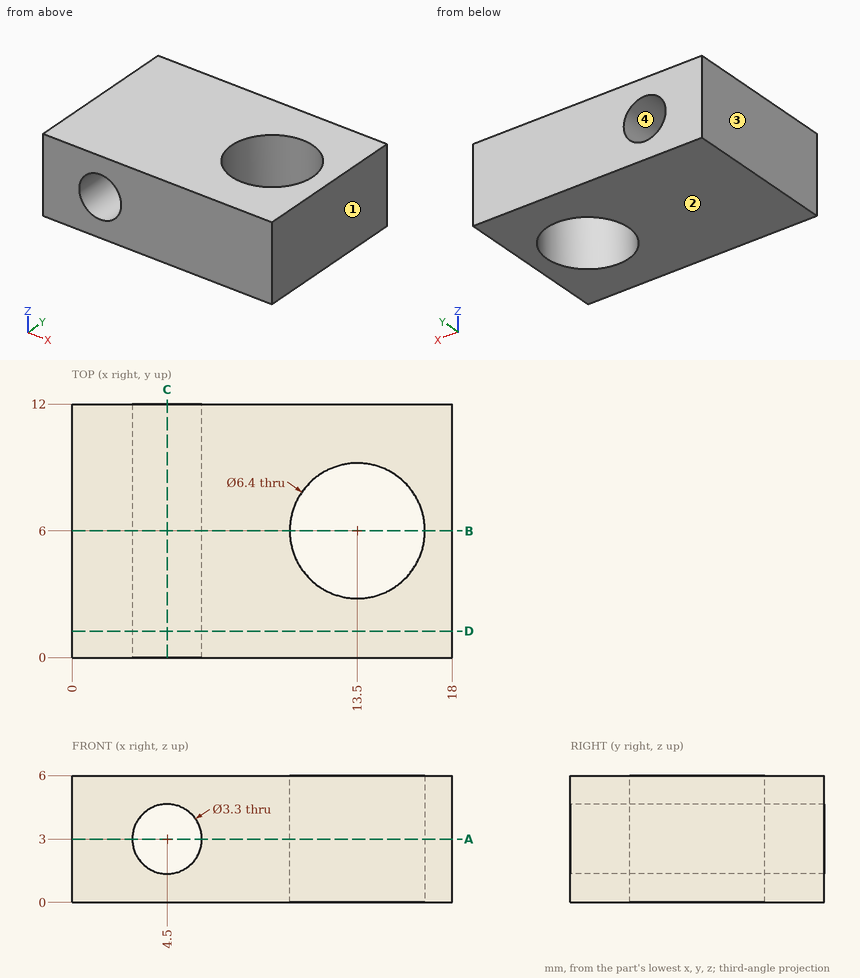
Could you check a few things on this drawing? It's one solid part, dimensions in mm from its lowest x, y, z. Coordinates: 2 decimals unless noted, no trailing zeros. Order: outer loops, then holes, each group sorted by start corner. A loop starts at its lowest first (then second) coordinate and runs counter-clockwise, first axis right, second up. Notation, with made-up numbers: (41.25, 64) - (59.25, 64) arc R22 cw to (59.25, 83) - close; hole circle Ø8 at (52.5, 64.5). An arc over 180 degrees is marked (long way). One line per question, with ' | ' between items. Start each with the question number.
1. If we mould it in two halves opening along X, with no side actions, what happens to the marked faces 1, 2, 3 and 4? For each: released by +X, released by -X, zero draft, split by the parting line, or undercut.
2. I'm going to push a flat-ended pin straight in: pin 1 Ø4 at (x, y) = (13, 5.5) entering from +Z. Where does the tip first touch, or does it pass through?
3. If we section it at D-D (y = 1.25): Write out the boundary of the cut face in (x, z).
4. If we section it at B-B (y = 6): Write out the boundary of the cut face in (x, z).
5. Please list where these lines run through material, in increasing order: line 1 along Y through (x, z) = (13.5, 2.6); line 2 along Z through (x, y) = (4.5, 2.75); line 3 along X through (y, z) = (5.5, 2.9). Write a range as [from, to].
6. If we section it at C-C (x = 4.5): Write out the boundary of the cut face in (y, z), and give its area (3 significant figures).
7. If we section it at A-A (z = 3): Write out the boundary of the cut face in (x, y).
Model answer:
1) face 1: released by +X | face 2: zero draft | face 3: released by -X | face 4: undercut
2) pin 1: passes through
3) outline: (0, 0) - (18, 0) - (18, 6) - (0, 6) - close; hole circle Ø3.3 at (4.5, 3)
4) outline: (0, 0) - (10.3, 0) - (10.3, 6) - (0, 6) - close; (16.7, 0) - (18, 0) - (18, 6) - (16.7, 6) - close; hole circle Ø3.3 at (4.5, 3)
5) line 1: y = [0, 2.8], [9.2, 12] | line 2: z = [0, 1.35], [4.65, 6] | line 3: x = [0, 2.85], [6.15, 10.34], [16.66, 18]
6) outline: (0, 0) - (12, 0) - (12, 1.35) - (0, 1.35) - close; (0, 4.65) - (12, 4.65) - (12, 6) - (0, 6) - close | area: 32.4 mm²
7) outline: (0, 0) - (2.85, 0) - (2.85, 12) - (0, 12) - close; (6.15, 0) - (18, 0) - (18, 12) - (6.15, 12) - close; hole circle Ø6.4 at (13.5, 6)
